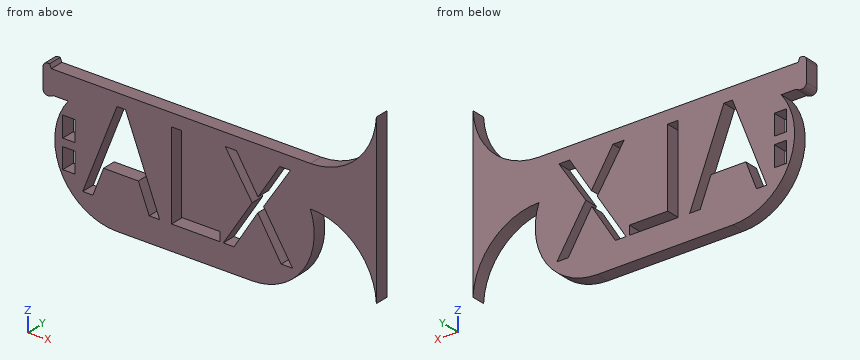
from build123d import *

# Parameters (mm, degrees)
F0_W     = 2.7374038473
F0_H     = 4.5464726281
F1_DEPTH = 3


with BuildPart() as f1:
    # F0 (on Front) → F1 (new body)
    with BuildSketch(Plane.XZ):
        with BuildLine():
            Line((-13.9879264009, 8.4983842463), (-10.7078288449, 8.4983842463))
            ThreePointArc((-10.7078288449, 8.4983842463), (-12.3096819162, -5.9457433928), (0, -13.6704108706))
            Line((0, -13.6704108706), (29.832560569, -13.6704108706))
            ThreePointArc((29.832560569, -13.6704108706), (41.0439649972, -7.8220549805), (42.6626390029, 4.7190275219))
            ThreePointArc((42.6626390029, 4.7190275219), (52.7277631814, 0.6811115523), (57.2114773095, -9.193492122))
            Line((57.2114773095, -9.193492122), (57.2114773095, 27.5829305145))
            ThreePointArc((57.2114773095, 27.5829305145), (52.7277631814, 17.7083268402), (42.6626390029, 13.6704108706))
            Line((42.6626390029, 13.6704108706), (29.832560569, 13.6704108706))
            Line((29.832560569, 13.6704108706), (0, 13.6704108706))
            Line((0, 13.6704108706), (-14.4307379611, 13.6704108706))
            Line((-14.4307379611, 13.6704108706), (-14.8297163701, 14.5122008398))
            Line((-14.8297163701, 14.5122008398), (-15.268201828, 14.5122008398))
            ThreePointArc((-15.268201828, 14.5122008398), (-15.9753086092, 14.219307621), (-16.268201828, 13.5122008398))
            Line((-16.268201828, 13.5122008398), (-16.268201828, 9.0994058373))
            ThreePointArc((-16.268201828, 9.0994058373), (-15.9753086092, 8.3922990562), (-15.268201828, 8.0994058373))
            Line((-15.268201828, 8.0994058373), (-14.8297163701, 8.0994058373))
            Line((-14.8297163701, 8.0994058373), (-13.9879264009, 8.4983842463))
        make_face()
        with Locations((-10.5523099191, -3.12910098)):
            Rectangle(F0_W, F0_H, mode=Mode.SUBTRACT)
        Polygon((9.4438036352, -8.2694776356), (7.1393343615, -8.2694776356), (4.7552561492, -2.1814888088), (-2.9165315603, -2.1814888088), (-5.2712801637, -8.2694776356), (-7.5254701078, -8.2694776356), (0.0415689984, 10.9539860515), (1.9144740263, 10.9539860515), align=None, mode=Mode.SUBTRACT)
        with Locations((-10.5523099191, 3.0826488801)):
            Rectangle(F0_W, F0_H, mode=Mode.SUBTRACT)
        Polygon((22.7468762609, -8.2694776356), (12.0750885514, -8.2694776356), (12.0750885514, 10.874377113), (14.2999488866, 10.874377113), (14.2999488866, -6.2541145071), (22.7468762609, -6.2541145071), align=None, mode=Mode.SUBTRACT)
        Polygon((32.3460382721, 1.811527951), (38.7357030766, -8.2694776356), (36.2091667637, -8.2694776356), (31.0639153671, 0.1481201297), (25.8264851995, -8.2694776356), (23.467546652, -8.2694776356), (29.8320717916, 1.7361089566), (23.8991108978, 10.874377113), (26.3627980486, 10.874377113), (31.1141946967, 3.2905782303), (35.9074907861, 10.874377113), (38.2748092218, 10.874377113), align=None, mode=Mode.SUBTRACT)
    extrude(amount=F1_DEPTH)


solid = f1.part
Read the model definition and answer for the solid it produces. Units are mm, in the model's axes. Give positions to 0.01 mm unless a question says otherwise; leave off trailing zeros. Write each loop counter-clockwise with the first axis right and the second up, starting at its lowest first coordinate (ties: lowest second). Pieces come first, ordered by that corner, then holes. Notation, with made-up numbers: (69, 8.25) - (76, 8.25) arc R27 cw to (76, 33.25) - close; hole circle Ø9 at (53, 56). An arc over 180 degrees is marked (long way). Answer in a Markdown table with one row per item. Add a question column.
Item 1: Flat-ended cylindrical pins translate along their axes: P1, Ø0.9, axis at x = 16.5, y = -2, coming from the +Z side; P2, Ø0.6, axis at y = -2, z = -7, coming from the -X side. Find the tip coordinate at first contact, or state that the pin passes through.
Item 2: Find the intervals of material crossed by L1, parallel to Z at x = 14, y = -1.5; L2, parallel to Z at x = 19, y = -2.8; L3, parallel to Z at x = -11, y = -0.25, in increasing order.
Item 3: Section D-D, the plane y = -1.7 is taken. Count the separate pieces of the cut face and the enclosed holes in it, and give its area (3 significant figures).
Item 4: Section B-B, the plane z = 6.5 is taken. Write down the section's boundary in (x, y), and give its area (3 significant figures).
Item 5: Section A-A, the plane x = 19.5 is taken. Write down the section's boundary in (y, z).
Item 6: Section C-C, the plane x = -6 is taken. Write down the section's boundary in (y, z).
Recorded:
| question | item | result |
|---|---|---|
| 1 | P1 | stops at z = 13.67 |
| 1 | P2 | stops at x = -11.92 |
| 2 | L1 | z = -13.67 to -8.27, 10.87 to 13.67 |
| 2 | L2 | z = -13.67 to -8.27, -6.25 to 13.67 |
| 2 | L3 | z = -8.12 to -5.4, -0.86 to 0.81, 5.36 to 8.12, 8.5 to 13.67 |
| 3 | separate pieces | 1 |
| 3 | enclosed holes | 5 |
| 3 | area | 1,410 mm2 |
| 4 | outline | (-12.03, -3) - (-1.71, -3) - (-1.71, 0) - (-12.03, 0) - close; (3.66, -3) - (12.08, -3) - (12.08, 0) - (3.66, 0) - close; (14.3, -3) - (26.74, -3) - (26.74, 0) - (14.3, 0) - close; (29.1, -3) - (33.14, -3) - (33.14, 0) - (29.1, 0) - close; (35.41, -3) - (57.21, -3) - (57.21, 0) - (35.41, 0) - close |
| 4 | area | 171 mm2 |
| 5 | outline | (-3, -13.67) - (0, -13.67) - (0, -8.27) - (-3, -8.27) - close; (-3, -6.25) - (0, -6.25) - (0, 13.67) - (-3, 13.67) - close |
| 6 | outline | (-3, -12.28) - (0, -12.28) - (0, -8.27) - (-3, -8.27) - close; (-3, -4.39) - (0, -4.39) - (0, 13.67) - (-3, 13.67) - close |
